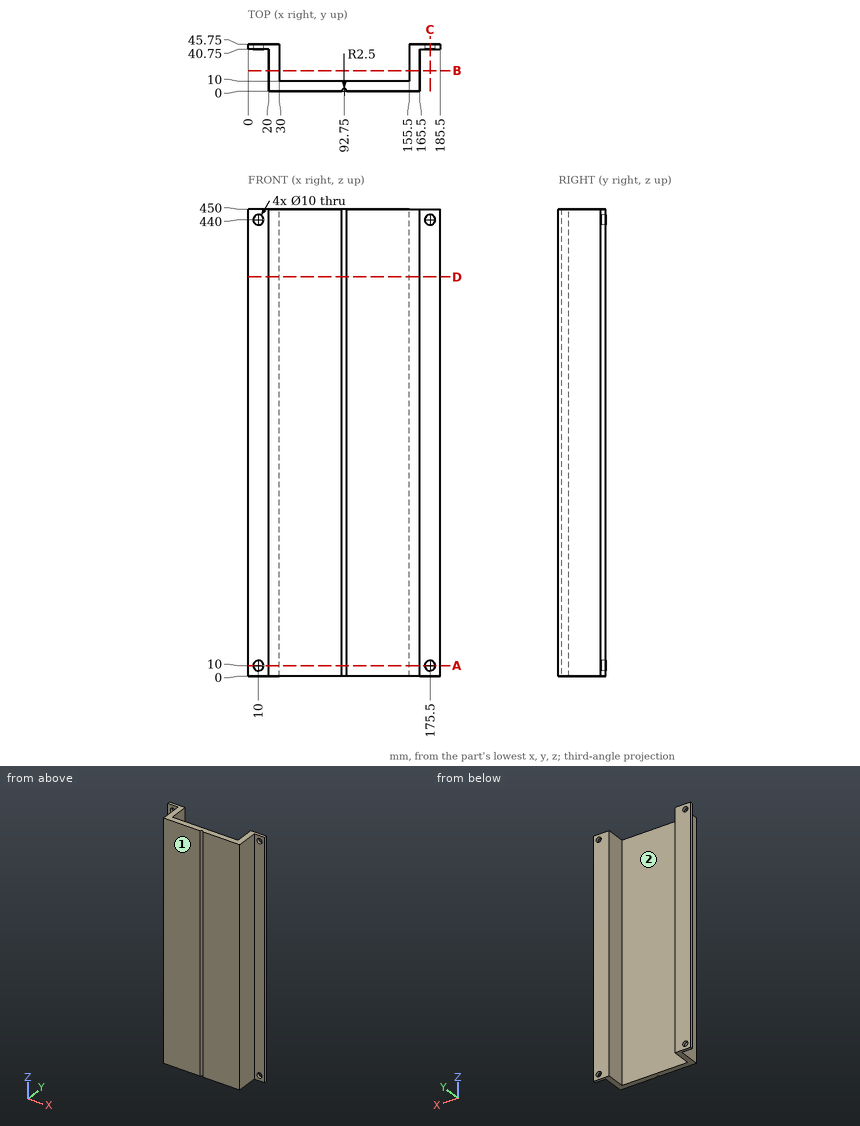
The drawing under review shows one solid part. Ordinate dimensions are in mm from its lowest x, y, z. Coordinates: 2 decimals unless noted, no trailing zeros. Loops run counter-clockwise (first coordinate to the right, second up) from the corner with the lowest first, then second, coordinate; pieces in that order, holes last. Notation, with made-up numbers: (-20, 4) -> (-1, 4) arc R17 cw to (-1, 19) -> close; hole circle Ø3 at (0, -14). An arc over 180 degrees is marked (long way). Answer as a JSON object with one key per item and string values.
Q1. The part is to be moulded in two halves that separate along X. For the marked faces 1 and 2, say which applies: +X half, -X half, draft (parallel to the pull), parting line (faces both ways), or undercut.
Answer block:
{"face 1": "draft", "face 2": "undercut"}
Q2. Clearance check with flat-ended pins moving along their axes: pin 1 Ø9 at (x, z) = (10, 10) entering from -Y; pin 2 Ø10 at (y, z) = (35.5, 121) entering from +X; pin 3 Ø3 at (x, z) = (143, 111.5) entering from +Y; pin 4 Ø22 at (x, z) = (7.5, 322.5) entering from -Y. State where each tip first meets the part, or that it passes through.
Answer block:
{"pin 1": "passes through", "pin 2": "stops at x = 165.5", "pin 3": "stops at y = 10", "pin 4": "stops at y = 40.75"}
Q3. Take a section at D-D on z = 385. Give the boundary of the cut face in (x, y), plus the area to 3 significant figures.
Answer block:
{"outline": "(0, 40.75) -> (20, 40.75) -> (20, 0) -> (90.25, 0) arc R2.5 cw to (95.25, 0) -> (165.5, 0) -> (165.5, 40.75) -> (185.5, 40.75) -> (185.5, 45.75) -> (155.5, 45.75) -> (155.5, 10) -> (30, 10) -> (30, 45.75) -> (0, 45.75) -> close", "area": "2,360 mm^2"}
Q4. Take a section at C-C on x = 175.5. Give the boundary of the cut face in (y, z).
Answer block:
{"outline": "(40.75, 0) -> (45.75, 0) -> (45.75, 5) -> (40.75, 5) -> close; (40.75, 15) -> (45.75, 15) -> (45.75, 435) -> (40.75, 435) -> close; (40.75, 445) -> (45.75, 445) -> (45.75, 450) -> (40.75, 450) -> close"}
Q5. To check wall thickness, follow L1, parallel to X at y = 44.2, z = 440; L2, parallel to Z at x = 10, y = 41.9; L3, parallel to X at y = 24, z = 69. State the ranges of each line that lie inside material, in increasing order.
Answer block:
{"L1": "x = 0 to 5, 15 to 30, 155.5 to 170.5, 180.5 to 185.5", "L2": "z = 0 to 5, 15 to 435, 445 to 450", "L3": "x = 20 to 30, 155.5 to 165.5"}
Q6. Take a section at A-A on z = 10. Give the boundary of the cut face in (x, y), plus the area to 3 significant figures.
Answer block:
{"outline": "(0, 40.75) -> (5, 40.75) -> (5, 45.75) -> (0, 45.75) -> close; (15, 40.75) -> (20, 40.75) -> (20, 0) -> (90.25, 0) arc R2.5 cw to (95.25, 0) -> (165.5, 0) -> (165.5, 40.75) -> (170.5, 40.75) -> (170.5, 45.75) -> (155.5, 45.75) -> (155.5, 10) -> (30, 10) -> (30, 45.75) -> (15, 45.75) -> close; (180.5, 40.75) -> (185.5, 40.75) -> (185.5, 45.75) -> (180.5, 45.75) -> close", "area": "2,260 mm^2"}
Q7. Take a section at B-B on y = 20. Give the boundary of the cut face in (x, z).
Answer block:
{"outline": "(20, 0) -> (30, 0) -> (30, 450) -> (20, 450) -> close; (155.5, 0) -> (165.5, 0) -> (165.5, 450) -> (155.5, 450) -> close"}
